from build123d import *

# Parameters (mm, degrees)
IZIM1_W                     = 30
IZIM1_H                     = 30
IZIM1_R                     = 2.25
Y_KSEKLIK_EKSTR_ZYON1_DEPTH = 10
RADYUS1_R                   = 3
IZIM2_R                     = 7
Y_KSEKLIK_EKSTR_ZYON2_DEPTH = 10
Y_KSEKLIK_EKSTR_ZYON2_TAPER = 5
IZIM3_R                     = 4.5
KES_EKSTR_ZYON1_DEPTH       = 30.154759474
KES_S_P_R2_PROFILE_R        = 1
KES_EKSTR_ZYON2_DEPTH       = 24.452078842
KES_EKSTR_ZYON2_DEPTH_BACK  = 4
IZIM34_R                    = 3.5


with BuildPart() as part:
    # Çizim1 → Yükseklik-Ekstrüzyon1 (new body)
    with BuildSketch(Plane.YZ):
        Rectangle(IZIM1_W, IZIM1_H)
        with Locations(Location((-7.071067812, 7.071067812, 0), (0, 0, 270))):
            Circle(IZIM1_R, mode=Mode.SUBTRACT)
        with Locations(Location((7.071067812, 7.071067812, 0), (0, 0, 270))):
            Circle(IZIM1_R, mode=Mode.SUBTRACT)
        with Locations(Location((7.071067812, -7.071067812, 0), (0, 0, 270))):
            Circle(IZIM1_R, mode=Mode.SUBTRACT)
        with Locations(Location((-7.071067812, -7.071067812, 0), (0, 0, 270))):
            Circle(IZIM1_R, mode=Mode.SUBTRACT)
    extrude(amount=Y_KSEKLIK_EKSTR_ZYON1_DEPTH)

    # Radyus1
    radyus1_edges = [part.edges().sort_by_distance(p)[0] for p in [
        (5, -15, 15),
        (5, 15, 15),
        (5, 15, -15),
        (5, -15, -15),
    ]]
    fillet(radyus1_edges, radius=RADYUS1_R)

    # Çizim2 → Yükseklik-Ekstrüzyon2 (add)
    with BuildSketch(Plane.YZ.offset(10)):
        Circle(IZIM2_R)
    extrude(amount=Y_KSEKLIK_EKSTR_ZYON2_DEPTH, taper=Y_KSEKLIK_EKSTR_ZYON2_TAPER)

    # Çizim3 → Kes-Ekstrüzyon1 (cut, through all)
    with BuildSketch(Plane.YZ.offset(20)):
        with Locations(Location((0, 0, 0), (0, 0, 270))):
            Circle(IZIM3_R)
    extrude(amount=-KES_EKSTR_ZYON1_DEPTH, mode=Mode.SUBTRACT)

    # Kes-Süpür2: sweep along a path in Çizim4
    with BuildLine(Plane(origin=(0.8, 0, 0), x_dir=(0, -1, 0), z_dir=(-1, 0, 0))) as kes_s_p_r2_path:
        Line((13, -12), (13, 12))
        ThreePointArc((13, 12), (12.707106781, 12.707106781), (12, 13))
        Line((12, 13), (-12, 13))
        ThreePointArc((-12, 13), (-12.707106781, 12.707106781), (-13, 12))
        Line((-13, 12), (-13, -12))
        ThreePointArc((-13, -12), (-12.707106781, -12.707106781), (-12, -13))
        Line((-12, -13), (12, -13))
        ThreePointArc((12, -13), (12.707106781, -12.707106781), (13, -12))
    # Kes-Süpür2 profile (on start of the path) → Kes-Süpür2 (sweep, cut)
    with BuildSketch(Plane(origin=(0.8, -13, -12), x_dir=(1, 0, 0), z_dir=(0, 0, 1))):
        Circle(KES_S_P_R2_PROFILE_R)
    sweep(path=kes_s_p_r2_path.line, mode=Mode.SUBTRACT)

    # Çizim34 → Kes-Ekstrüzyon2 (cut, two sides: drawn at the far end of the back side and taken through both)
    with BuildSketch(Plane.YZ.offset(10).offset(-KES_EKSTR_ZYON2_DEPTH_BACK)):
        with Locations(Location((-7.071067812, 7.071067812, 0), (0, 0, 340.368439442))):
            Circle(IZIM34_R)
        with Locations(Location((7.071067812, 7.071067812, 0), (0, 0, 199.631561315))):
            Circle(IZIM34_R)
        with Locations(Location((7.071067812, -7.071067812, 0), (0, 0, 109.631561315))):
            Circle(IZIM34_R)
        with Locations(Location((-7.071067812, -7.071067812, 0), (0, 0, 70.368439442))):
            Circle(IZIM34_R)
    extrude(amount=KES_EKSTR_ZYON2_DEPTH + KES_EKSTR_ZYON2_DEPTH_BACK, mode=Mode.SUBTRACT)


solid = part.part
Could you check a few things on this model? Use its own coordinates, in mm. A direction names the side the tool comes from. Coordinates: 2 decimals unless noted, no trailing zeros. Write each loop counter-clockwise with the first axis right and the second up, starting at its lowest first coordinate (ties: lowest second). Pieces come first, ordered by that corner, then holes. Notation, with made-up numbers: (-19, -13) - (4, -13) arc R22 ccw to (4, 9) - close; hole circle Ø8 at (10.25, -34). An arc over 180 degrees is marked (long way). Put each result on its own line as item: value. Start each with the question number.
Q1. Which directions (+Z, -Z, +X, -X, +Y, -Y) give clear straight access to the entire face, cutting with the end or side of a thin tool? Please do faces 1 (the flat face through (6, -4.67, -7.15)), 2 (the cylindrical face through (1.8, 13, -0.2)), 3 (the flat face through (0, -1, -14)).
Q2. I want a section at B-B on x = 9. Write out the boundary of the cut face in (y, z), plus the area to 3 significant figures.
Q3. Thinking about a two-plate mould opening in X: for faces 4 (the cylindrical face through (1.8, -0.2, -13)), 5 (the cylindrical face through (1.8, 0.2, 13)), 6 (the flat face through (0, 5, 0)), 7 (the cylindrical face through (2.96, -6.4, -9.22)), which applies, pulls with the +X half, pulls with the -X half, needs draft (parallel to the pull), parting line crosses it, or undercut?
Q4. I want a section at C-C on y = 7.75. Write out the boundary of the cut face in (x, z).
Q5. I'm going to push flat-ended pins straight in: P1, Ø4, axis at y = -9, z = 5, coming from the +X side; P2, Ø5, axis at y = 7.07, z = -7.07, coming from the +X side; P3, Ø1.5, axis at x = 16, y = 6.5, coming from the -Z side. Where does each tip first touch, or does it pass through?
Q6. Please list where these lines run through material, in increasing order: L1, parallel to Z at x = 0.8, y = -2.25; L2, parallel to Y at x = 8.25, z = -10.25; L3, parallel to Y at x = 1, z = 2.
Q7. I want a section at A-A on y = 0. Write out the boundary of the cut face in (x, z), plus the area to 3 significant figures.
Checks:
1. face 1: +X
1. face 2: none
1. face 3: +Z, -Z, -X, +Y, -Y
2. outline: (-15, -12) arc R3 ccw to (-12, -15) - (12, -15) arc R3 ccw to (15, -12) - (15, 12) arc R3 ccw to (12, 15) - (-12, 15) arc R3 ccw to (-15, 12) - close; hole circle Ø7 at (-7.07, -7.07); hole circle Ø7 at (-7.07, 7.07); hole circle Ø9 at (0, 0); hole circle Ø7 at (7.07, -7.07); hole circle Ø7 at (7.07, 7.07)
2. area: 675 mm²
3. face 4: undercut
3. face 5: undercut
3. face 6: pulls with the -X half
3. face 7: needs draft
4. outline: (0, -15) - (10, -15) - (10, -10.5) - (6, -10.5) - (6, -9.22) - (0, -9.22) - (0, -12.4) arc R1 cw (long way) to (0, -13.6) - close; (0, -4.93) - (6, -4.93) - (6, -3.64) - (10, -3.64) - (10, 3.64) - (6, 3.64) - (6, 4.93) - (0, 4.93) - close; (0, 9.22) - (6, 9.22) - (6, 10.5) - (10, 10.5) - (10, 15) - (0, 15) - (0, 13.6) arc R1 cw (long way) to (0, 12.4) - close
5. P1: x = 10
5. P2: x = 6
5. P3: z = -2.98
6. L1: -15 to -14, -12 to -3.9, 3.9 to 12, 14 to 15
6. L2: -15 to -8.54, -5.61 to 5.61, 8.54 to 15
6. L3: -15 to -13.98, -12.02 to -4.03, 4.03 to 12.02, 13.98 to 15
7. outline: (0, -15) - (10, -15) - (10, -7) - (20, -6.13) - (20, -4.5) - (0, -4.5) - (0, -12.4) arc R1 cw (long way) to (0, -13.6) - close; (0, 4.5) - (20, 4.5) - (20, 6.13) - (10, 7) - (10, 15) - (0, 15) - (0, 13.6) arc R1 cw (long way) to (0, 12.4) - close
7. area: 245 mm²
